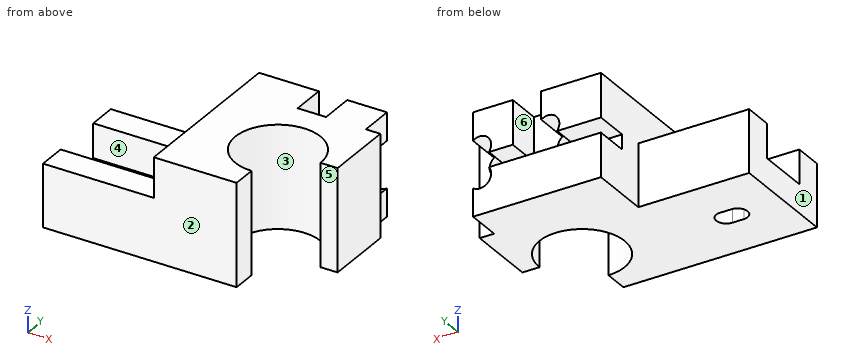
```python
from build123d import *

# Parameters (mm, degrees)
SKETCH1_W               = 8.56892
SKETCH1_H               = 8.11892
BOSS_EXTRUDE1_DEPTH     = 9
SKETCH4_W               = 19.5
SKETCH4_H               = 19.25
BOSS_EXTRUDE2_DEPTH     = 5
SKETCH5_W               = 19.5
SKETCH5_H               = 5
BOSS_EXTRUDE3_DEPTH     = 6
CUT_EXTRUDE1_DEPTH      = 6
SKETCH7_R               = 2
CUT_EXTRUDE2_DEPTH      = 10
CUT_EXTRUDE3_DEPTH      = 6
SKETCH11_R              = 7.5
SKETCH11_W              = 10.5
SKETCH11_H              = 11.73108
CUT_EXTRUDE5_DEPTH      = 10
CUT_EXTRUDE5_DEPTH_BACK = 10


with BuildPart() as part:
    # Sketch1 → Boss-Extrude1 (new body, symmetric)
    with BuildSketch(Plane.XY):
        Polygon((-16.5, -19.85), (0, -19.85), (0, 0), (8.56892, 0), (8.56892, 10), (-16.5, 10), align=None)
        with Locations((4.28446, -4.05946)):
            Rectangle(SKETCH1_W, SKETCH1_H)
    extrude(amount=BOSS_EXTRUDE1_DEPTH, both=True)

    # Sketch4 → Boss-Extrude2 (add)
    with BuildSketch(Plane(origin=(0, 0, -9), x_dir=(-1, 0, 0), z_dir=(0, 0, -1))):
        with Locations((26.25, -10.225)):
            Rectangle(SKETCH4_W, SKETCH4_H)
    extrude(amount=-BOSS_EXTRUDE2_DEPTH)

    # Sketch5 → Boss-Extrude3 (add)
    with BuildSketch(Plane.XY.offset(-4)):
        with Locations((-26.25, -17.35)):
            Rectangle(SKETCH5_W, SKETCH5_H)
        with Locations((-26.25, -3.1)):
            Rectangle(SKETCH5_W, SKETCH5_H)
    extrude(amount=BOSS_EXTRUDE3_DEPTH)

    # Sketch6 → Cut-Extrude1 (cut)
    with BuildSketch(Plane.XY.offset(-4)):
        with BuildLine():
            Line((-28, -8.475), (-26, -8.475))
            ThreePointArc((-26, -8.475), (-24.25, -10.225), (-26, -11.975))
            Line((-26, -11.975), (-28, -11.975))
            ThreePointArc((-28, -11.975), (-29.75, -10.225), (-28, -8.475))
        make_face()
    extrude(amount=-CUT_EXTRUDE1_DEPTH, mode=Mode.SUBTRACT)

    # Sketch7 → Cut-Extrude2 (cut)
    with BuildSketch(Plane(origin=(0, 10, 0), x_dir=(1, 0, 0), z_dir=(0, 1, 0))):
        with Locations((4.81892, 2.5)):
            Circle(SKETCH7_R)
        with Locations((4.81892, -2.5)):
            Circle(SKETCH7_R)
        with Locations((-7.18108, -2.5)):
            Circle(SKETCH7_R)
    extrude(amount=-CUT_EXTRUDE2_DEPTH, mode=Mode.SUBTRACT)

    # Sketch8 → Cut-Extrude3 (cut)
    with BuildSketch(Plane(origin=(0, 10, 0), x_dir=(1, 0, 0), z_dir=(0, 1, 0))):
        Polygon((6.01892, 1.3), (6.01892, 9), (8.56892, 9), (8.56892, -9), (6.01892, -9), (6.01892, -1.3), (-0.98108, -1.3), (-0.98108, -9), (-5.98108, -9), (-5.98108, -1.3), (-16.5, -1.3), (-16.5, 1.3), align=None)
    extrude(amount=-CUT_EXTRUDE3_DEPTH, mode=Mode.SUBTRACT)

    # Sketch11 → Cut-Extrude5 (cut, two sides)
    with BuildSketch(Plane.XY) as cut_extrude5_sk:
        with Locations((-1.93108, -8.11892)):
            Circle(SKETCH11_R)
        with Locations((3.31892, -13.98446)):
            Rectangle(SKETCH11_W, SKETCH11_H)
    extrude(amount=CUT_EXTRUDE5_DEPTH, mode=Mode.SUBTRACT)
    extrude(cut_extrude5_sk.sketch, amount=-CUT_EXTRUDE5_DEPTH_BACK, mode=Mode.SUBTRACT)


solid = part.part
```
Geometry: final body of the model. Coordinates: model frame, mm. Face numbers are marked on the shaded views. A direction names the side the tool comes from. Give positions to 0.01 mm unless a question says otherwise; leave off trailing zeros. Loops run counter-clockwise (first coordinate to the right, second up) from the corner with the lowest first, then second, coordinate; pieces in that order, holes last. Notation, with made-up numbers: (43.5, 68) - (56.5, 68) arc R18 cw to (56.5, 96) - close; hole circle Ø5 at (-23, 47). An arc over 180 degrees is marked (long way). Answer as CSV lines item,"result". Start each with the question number.
(1) Section query D-D (x = -2.5). Output: boundary loops of the cut face in (y, z), and give its area (3 significant figures).
(2) Section query B-B (y = -11.25). Output: boundary loops of the cut face in (x, z).
(3) Pin query (flat end, axial travel): P1, Ø5, axis at x = -17, y = -10.5, coming from the +Z side; P2, Ø8, axis at y = 6, z = 4, coming from the -X side; P3, Ø1.3, axis at y = -18, z = -4.5, coming from the +X side; P4, Ø2, axis at x = 5.5, z = 2.5, coming from the +Y side. Return the tip coordinate at first contact, or that it passes through.
(4) Ray query, line 1 along X through (y, z) = (3.75, 2.5); line 2 along X through (y, z) = (2.75, -2.5); line 3 along Z through (x, y) = (0, 6). Return the intervals inside material, ascending. Write a range as [from, to].
(5) Section query A-A (z = 2.5). Output: boundary loops of the cut face in (x, y).
(6) Section query C-C (x = -17). Output: boundary loops of the cut face in (y, z), and give its area (3 significant figures).
(7) Reachability of the marked faces 4, 5 and 6 from +Z, -Z, +X, -X, +Y, -Y: full face, straight path, thin tool, end or side. Return the list, or none.
(8) Mould query, pull axis Y, two halves, no side actions, for the marked faces 1, 2 and 3. Classes: +Y half, -Y half, draft (parallel to the pull), parting line (faces both ways), or undercut.
Worked answers:
1,outline,"(-19.85, -9) - (-15.6, -9) - (-15.6, 9) - (-19.85, 9) - close; (-0.64, -9) - (10, -9) - (10, -1.3) - (4, -1.3) - (4, 9) - (-0.64, 9) - close"
1,area,"206 mm^2"
2,outline,"(-36, -9) - (-29.42, -9) - (-29.42, -4) - (-36, -4) - close; (-24.58, -9) - (-8.75, -9) - (-8.75, 9) - (-16.5, 9) - (-16.5, -4) - (-24.58, -4) - close"
3,P1,"stops at z = 9"
3,P2,"stops at x = -16.5"
3,P3,"stops at x = -1.93"
3,P4,"stops at y = 0"
4,line 1,"x = [-16.5, -9.18], [-5.18, 2.82], [6.82, 8.57]"
4,line 2,"x = [-16.5, 2.82], [6.82, 8.57]"
4,line 3,"z = [-9, -1.3], [1.3, 9]"
5,outline,"(-16.5, -19.85) - (-1.93, -19.85) - (-1.93, -15.62) arc R7.5 cw (long way) to (5.57, -8.12) - (8.57, -8.12) - (8.57, 4) - (6.82, 4) - (6.82, 0) - (2.82, 0) - (2.82, 10) - (-0.98, 10) - (-0.98, 4) - (-5.18, 4) - (-5.18, 0) - (-9.18, 0) - (-9.18, 10) - (-16.5, 10) - close"
6,outline,"(-19.85, -9) - (-0.6, -9) - (-0.6, 2) - (-5.6, 2) - (-5.6, -4) - (-14.85, -4) - (-14.85, 2) - (-19.85, 2) - close"
6,area,"156 mm^2"
7,face 4,"+Z, -X"
7,face 5,"+Z, -Z, +X, -Y"
7,face 6,"+Z, +Y"
8,face 1,"draft"
8,face 2,"-Y half"
8,face 3,"undercut"
